Here's the drawing with two shaded views (mm, measured from the low corner). I have some questions. A direction names the side the tool comes from. Give positions to 0.01 mm unless a question says otherwise; leave off trailing zeros. Loops run counter-clockwise (first coordinate to the right, second up) from the corner with the lowest first, then second, coordinate; pieces in that order, holes last. Notation, with made-up numbers: M 4,19.5 L 22,19.5 A20 cw 22,26.5 Z; hole C 35,-0.75 d8. An arc over 180 degrees is marked long. Use CSV: the item, a comma, the result in double quotes.
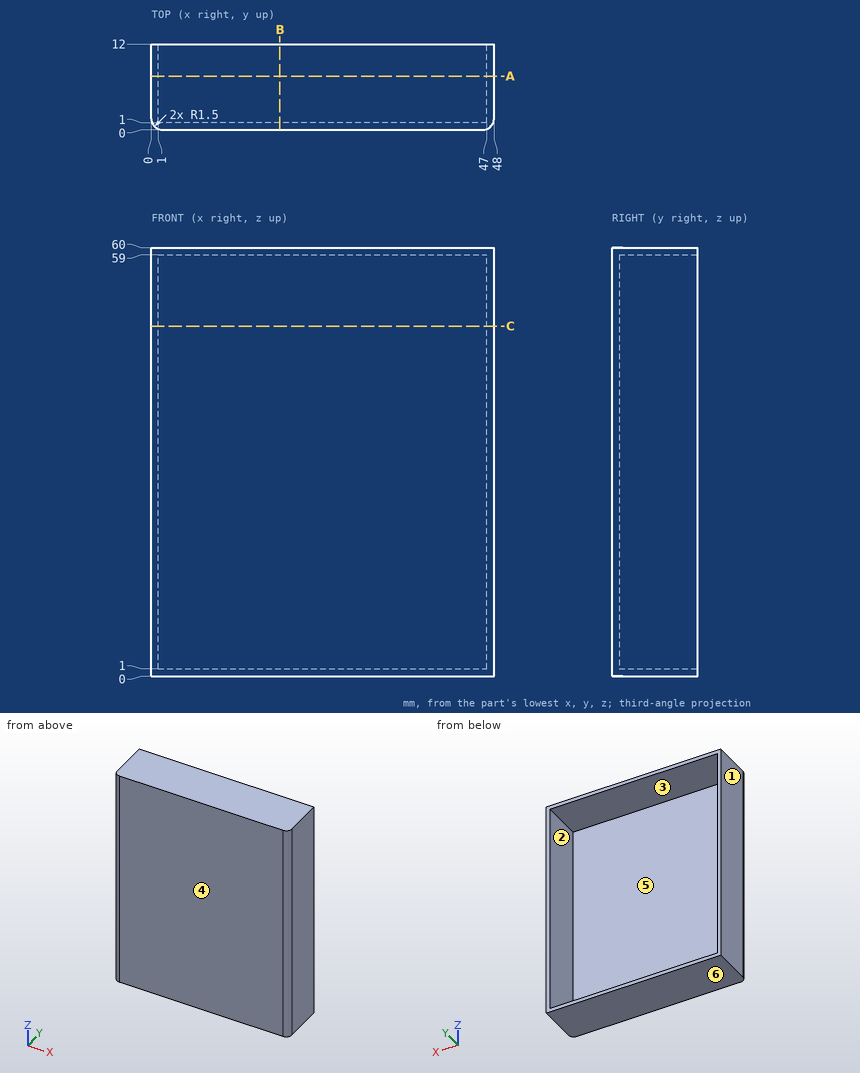
1. I want a section at A-A, the plane y = 7.5. List the corners of the cut face in (x, z) for me, then the cut area to 3 significant figures.
Outcome:
outline,"M 0,0 L 48,0 L 48,60 L 0,60 Z; hole M 1,1 L 47,1 L 47,59 L 1,59 Z"
area,"212 mm2"
2. Which directions (+Z, -Z, +X, -X, +Y, -Y) give clear straight access to the entire face, cutting with the end or side of a thin tool? Please do the marked faces 5 and 6.
Outcome:
face 5,"+Y"
face 6,"-Z, +X, -X, +Y, -Y"
3. I want a section at B-B, the plane x = 18. List the corners of the cut face in (y, z) for me.
Outcome:
outline,"M 0,0 L 12,0 L 12,1 L 1,1 L 1,59 L 12,59 L 12,60 L 0,60 Z"
4. I want a section at C-C, the plane z = 49. List the corners of the cut face in (x, y) for me.
Outcome:
outline,"M 0,1.5 A1.5 ccw 1.5,0 L 46.5,0 A1.5 ccw 48,1.5 L 48,12 L 47,12 L 47,1 L 1,1 L 1,12 L 0,12 Z"
5. If we mould it in two halves opening along X, with no side actions, what happens to the marked faces 1, 2, 3 and 4? For each: +X half, -X half, draft (parallel to the pull), parting line (faces both ways), or undercut.
Outcome:
face 1,"-X half"
face 2,"undercut"
face 3,"undercut"
face 4,"draft"
6. Please list where these lines run through material, in increasing order: line 1 (Z direction, x = 30.5, y = 5.25); line 2 (X direction, y = 7.5, z = 44); line 3 (Y direction, x = 29, z = 34.5).
Outcome:
line 1,"0 to 1, 59 to 60"
line 2,"0 to 1, 47 to 48"
line 3,"0 to 1"
7. I'm going to push a flat-ended pin straight in: pin 1 Ø6 at (x, z) = (7, 45) entering from +Y. Where does the tip first touch, or does it pass through?
Outcome:
pin 1,"y = 1"
